Geometry check sheet. Reference: the model listing, model coordinates, mm. Face numbers are marked on the shaded views. A direction names the side the tool comes from. Round coordinates to 2 decimals unless told otherwise and drop trailing zeros. Order: outer loops, then holes, each group sorted by start corner. A loop starts at its lowest first (then second) coordinate and runs counter-clockwise, first axis right, second up. Notation, with made-up numbers: (69.25, 49.5) - (96.25, 49.5) arc R33 ccw to (96.25, 82.5) - close; hole circle Ø8 at (-27, 88.25). An arc over 180 degrees is marked (long way). Return JSON: item names as keys, results as strings. Group by question number.
Q1. Gauge pin test, flat ends, axial feed: pin 1 Ø4 at (y, z) = (2, 16) entering from -X; pin 2 Ø5 at (y, z) = (5.5, 12.5) entering from -X; pin 3 Ø10 at (x, z) = (-2.5, 17.5) entering from -Y. Record the tip position at first contact, or that the pin passes through.
Q2. Sectioned sample at A-A, the plane y = 0. Record the cut outline in (x, z).
Q3. Tool access check on the marked faces 1 and 2. Record the directions out of +Z, -Z, +X, -X, +Y, -Y that give a thin tool (end or side, any length) a straight path to the whole face; none if there is none.
Q4. Sectioned sample at D-D, the plane x = 6. Record the cut outline in (y, z), then the cut area to 3 significant figures.
Q5. Sectioned sample at C-C, the plane z = 27. Record the cut outline in (x, y), then the cut area to 3 significant figures.
Q6. Material ranges on line 1 along X through (y, z) = (0, 78); line 2 along Z through (x, y) = (4.5, 4), recorded low to high.
```python
from build123d import *

# Parameters (mm, degrees)
F0_R     = 8.5
F1_DEPTH = 4
F2_R     = 5
F3_DEPTH = 100
F4_W     = 4
F4_H     = 5
F6_R     = 1.5
F7_DEPTH = 90


with BuildPart() as f1:
    # F0 (on Top) → F1 (new body)
    with BuildSketch(Plane.XY):
        Circle(F0_R)
    extrude(amount=F1_DEPTH)

    # F2 (on Top) → F3 (join)
    with BuildSketch(Plane.XY):
        Circle(F2_R)
    extrude(amount=F3_DEPTH)

    # F4 (on Right) → F5 (revolve)
    with BuildSketch(Plane.YZ):
        with Locations((2, 102.5)):
            Rectangle(F4_W, F4_H)
    revolve(axis=Axis((0, 0, 102.5), (0, 0, -1)))

    # F6 (on face) → F7 (cut)
    with BuildSketch(Plane(origin=(0, 0, 0), x_dir=(1, 0, 0), z_dir=(0, 0, -1))):
        Circle(F6_R)
    extrude(amount=-F7_DEPTH, mode=Mode.SUBTRACT)


solid = f1.part
```
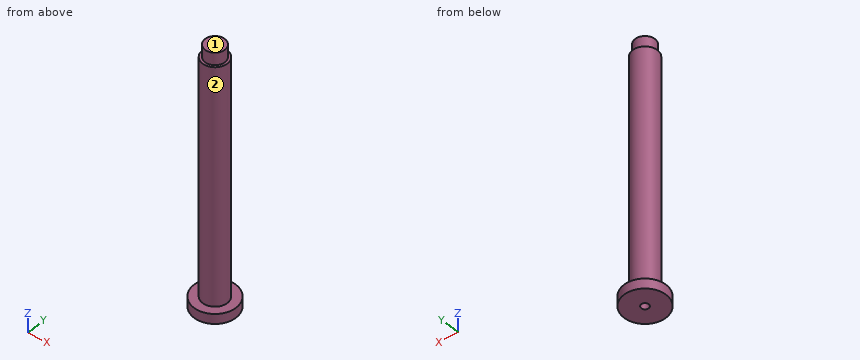
Reply:
{
 "1": {"pin 1": "x = -5", "pin 2": "x = -4", "pin 3": "y = -5"},
 "2": {"outline": "(-8.5, 0) - (-1.5, 0) - (-1.5, 90) - (1.5, 90) - (1.5, 0) - (8.5, 0) - (8.5, 4) - (5, 4) - (5, 100) - (4, 100) - (4, 105) - (-4, 105) - (-4, 100) - (-5, 100) - (-5, 4) - (-8.5, 4) - close"},
 "3": {"face 1": "+Z, +X, -X, +Y, -Y", "face 2": "+Z"},
 "4": {"outline": "(-6.02, 0) - (6.02, 0) - (6.02, 4) - (-6.02, 4) - close", "area": "48.2 mm^2"},
 "5": {"outline": "circle Ø10 at (0, 0); hole circle Ø3 at (0, 0)", "area": "71.5 mm^2"},
 "6": {"line 1": "-5 to -1.5, 1.5 to 5", "line 2": "0 to 4"}
}
